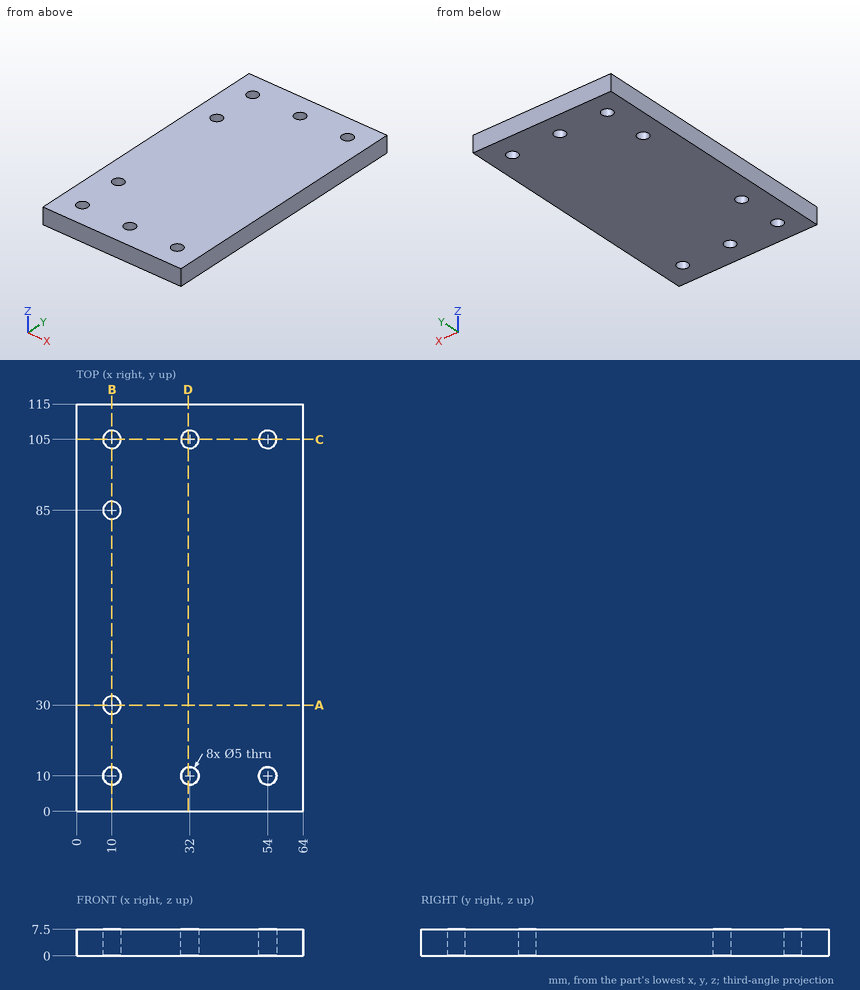
Here's the drawing with two shaded views (mm, measured from the low corner). I have some questions. Give positions to 0.01 mm unless a question says otherwise; leave off trailing zeros. Loops run counter-clockwise (first coordinate to the right, second up) from the corner with the lowest first, then second, coordinate; pieces in that order, holes last. Notation, with made-up numbers: M -3,38 L 16,38 A31 ccw 16,62 Z; hole C 30.25,4.5 d1. An arc over 180 degrees is marked long. One line per item, written item: value. Start each with the question number.
1) If we section it at B-B, the plane x = 10: Write out the boundary of the cut face in (y, z).
2) If I drill on line 1 (Y direction, x = 54, z = 3.5); line 2 (X direction, y = 105, z = 3.75); line 3 (Y direction, x = 10, z = 3), over which ranges is the centre line in solid material (lowest first)? Write a range as [from, to].
3) If we section it at A-A, the plane y = 30: Write out the boundary of the cut face in (x, z).
4) I'm going to push a flat-ended pin straight in: pin 1 (4.5 mm diameter, centred on x = 32, y = 105, fed in from +Z). Where does the tip first touch, or does it pass through?
5) If we section it at D-D, the plane x = 31.5: Write out the boundary of the cut face in (y, z), and give its area (3 significant figures).
6) If we section it at C-C, the plane y = 105: Write out the boundary of the cut face in (x, z), and give its area (4 significant figures).
Completed:
1. outline: M 0,0 L 7.5,0 L 7.5,7.5 L 0,7.5 Z; M 12.5,0 L 27.5,0 L 27.5,7.5 L 12.5,7.5 Z; M 32.5,0 L 82.5,0 L 82.5,7.5 L 32.5,7.5 Z; M 87.5,0 L 102.5,0 L 102.5,7.5 L 87.5,7.5 Z; M 107.5,0 L 115,0 L 115,7.5 L 107.5,7.5 Z
2. line 1: y = [0, 7.5], [12.5, 102.5], [107.5, 115]
2. line 2: x = [0, 7.5], [12.5, 29.5], [34.5, 51.5], [56.5, 64]
2. line 3: y = [0, 7.5], [12.5, 27.5], [32.5, 82.5], [87.5, 102.5], [107.5, 115]
3. outline: M 0,0 L 7.5,0 L 7.5,7.5 L 0,7.5 Z; M 12.5,0 L 64,0 L 64,7.5 L 12.5,7.5 Z
4. pin 1: passes through
5. outline: M 0,0 L 7.55,0 L 7.55,7.5 L 0,7.5 Z; M 12.45,0 L 102.55,0 L 102.55,7.5 L 12.45,7.5 Z; M 107.45,0 L 115,0 L 115,7.5 L 107.45,7.5 Z
5. area: 789 mm^2
6. outline: M 0,0 L 7.5,0 L 7.5,7.5 L 0,7.5 Z; M 12.5,0 L 29.5,0 L 29.5,7.5 L 12.5,7.5 Z; M 34.5,0 L 51.5,0 L 51.5,7.5 L 34.5,7.5 Z; M 56.5,0 L 64,0 L 64,7.5 L 56.5,7.5 Z
6. area: 367.5 mm^2
